Here's how the part is built. I have some questions about the finished solid (model axes, mm). Face numbers are marked on the shaded views. Coordinates: 2 decimals unless noted, no trailing zeros. Order: outer loops, then holes, each group sorted by start corner. A loop starts at its lowest first (then second) coordinate and runs counter-clockwise, first axis right, second up. Notation, with made-up numbers: (-12.5, 75.5) - (43.5, 75.5) arc R17 ccw to (43.5, 94.5) - close; hole circle Ø8 at (85.5, -22.75). An arc over 180 degrees is marked (long way). Answer as CSV lines item,"result". Start each with the question number.
Q1. Suppose I cut it at C-C (z = -35). Please give me the cut outline in (x, y).
Q2. Suppose I cut it at A-A (x = 0). Please give me the cut outline in (y, z), then the cut area to 3 significant figures.
Q3. For pin 1 Ø2.5 at (x, z) = (-23.57, 28.57) entering from +Y, with a flat end and sliding along its axis, tell me the tip position at first contact or that it passes through.
Q4. I need wall thicknesses on line 1 (Z direction, x = 23.57, y = -5.25); line 2 (X direction, y = -15, z = 28.57); line 3 (Z direction, x = 45, y = -11). Which ranges of each line are inside material? Lowest first, please.
Q5. Thinking about a two-plate mould opening in X: for the marked faces 1, 2 and 3, which applies, released by +X, released by -X, zero draft, split by the parting line, or undercut?
Q6. Suppose I cut it at B-B (y = -16.75). Count the separate pieces of the cut face and the enclosed holes in it, then the cut area to 3 significant figures.
Q7. Suppose I cut it at D-D (x = 97.5). Please give me the cut outline in (y, z).
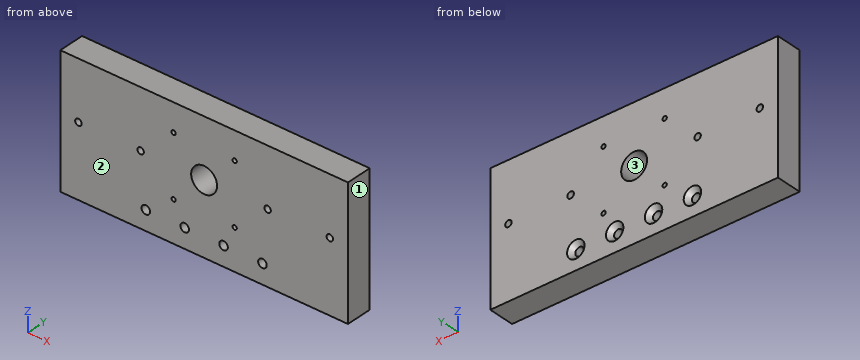
from build123d import *

# Parameters (mm, degrees)
F0_W           = 222
F0_H           = 100
F0_R           = 10
F1_DEPTH       = 20
F2_D           = 5
F3_D           = 6.6
F3_CSINK_D     = 13.44
F3_CSINK_ANGLE = 90
F4_D           = 3.3


with BuildPart() as f1:
    # F0 (on Front) → F1 (new body)
    with BuildSketch(Plane.XZ):
        Rectangle(F0_W, F0_H)
        with Locations((0, 5)):
            Circle(F0_R, mode=Mode.SUBTRACT)
    extrude(amount=F1_DEPTH)

    # F2 (through all)
    with Locations(Plane(origin=(0, 0, 0), x_dir=(1, 0, 0), z_dir=(0, 1, 0))):
        with Locations((49, -5), (97, -5), (-49, -5), (-97, -5)):
            Hole(F2_D / 2)

    # F3 (through all)
    with Locations(Plane(origin=(0, 0, 0), x_dir=(1, 0, 0), z_dir=(0, 1, 0))):
        with Locations((-45, 35), (-15, 35), (15, 35), (45, 35)):
            CounterSinkHole(F3_D / 2, F3_CSINK_D / 2, counter_sink_angle=F3_CSINK_ANGLE)

    # F4 (through all)
    with Locations(Plane(origin=(0, 0, 0), x_dir=(1, 0, 0), z_dir=(0, 1, 0))):
        with Locations((23.57, -28.57), (-23.57, -28.57), (23.57, 18.57), (-23.57, 18.57)):
            Hole(F4_D / 2)


solid = f1.part
Here are the results:
1,outline,"(-111, -20) - (-48.3, -20) - (-48.3, -3.42) - (-51.72, 0) - (-111, 0) - close; (-41.7, -20) - (-18.3, -20) - (-18.3, -3.42) - (-21.72, 0) - (-38.28, 0) - (-41.7, -3.42) - close; (-11.7, -20) - (11.7, -20) - (11.7, -3.42) - (8.28, 0) - (-8.28, 0) - (-11.7, -3.42) - close; (18.3, -20) - (41.7, -20) - (41.7, -3.42) - (38.28, 0) - (21.72, 0) - (18.3, -3.42) - close; (48.3, -20) - (111, -20) - (111, 0) - (51.72, 0) - (48.3, -3.42) - close"
2,outline,"(-20, -50) - (0, -50) - (0, -5) - (-20, -5) - close; (-20, 15) - (0, 15) - (0, 50) - (-20, 50) - close"
2,area,"1,600 mm²"
3,pin 1,"passes through"
4,line 1,"z = -50 to -20.22, -16.92 to 26.92, 30.22 to 50"
4,line 2,"x = -111 to -25.22, -21.92 to 21.92, 25.22 to 111"
4,line 3,"z = -50 to -38.3, -31.7 to 50"
5,face 1,"released by +X"
5,face 2,"zero draft"
5,face 3,"undercut"
6,separate pieces,"1"
6,enclosed holes,"13"
6,area,"21,600 mm²"
7,outline,"(-20, -50) - (0, -50) - (0, 2.55) - (-20, 2.55) - close; (-20, 7.45) - (0, 7.45) - (0, 50) - (-20, 50) - close"
